```python
from build123d import *

# Parameters (mm, degrees)
SKETCH1_R           = 2.3
BOSS_EXTRUDE2_DEPTH = 4
FILLET1_R           = 4
FILLET2_R           = 30


with BuildPart() as part:
    # Sketch1 → Boss-Extrude2 (new body)
    with BuildSketch(Plane(origin=(0, 0, 0), x_dir=(1, 0, 0), z_dir=(0, 1, 0))):
        with BuildLine():
            Line((-4, -143.7), (-4, 4))
            Line((-4, 4), (25.4, 4))
            ThreePointArc((25.4, 4), (28.6800532, 2.289377864), (29.154640594, -1.379374498))
            Line((29.154640594, -1.379374498), (4, -69.85))
            Line((4, -69.85), (29.154640594, -138.320625502))
            ThreePointArc((29.154640594, -138.320625502), (28.6800532, -141.989377864), (25.4, -143.7))
            Line((25.4, -143.7), (-4, -143.7))
        make_face()
        with Locations(Location((0, 0, 0), (0, 0, 270))):
            Circle(SKETCH1_R, mode=Mode.SUBTRACT)
        with Locations(Location((25.4, 0, 0), (0, 0, 270))):
            Circle(SKETCH1_R, mode=Mode.SUBTRACT)
        with Locations(Location((25.4, -139.7, 0), (0, 0, 270))):
            Circle(SKETCH1_R, mode=Mode.SUBTRACT)
        with Locations(Location((0, -139.7, 0), (0, 0, 270))):
            Circle(SKETCH1_R, mode=Mode.SUBTRACT)
    extrude(amount=BOSS_EXTRUDE2_DEPTH)

    # Fillet1
    fillet1_edges = [part.edges().sort_by_distance(p)[0] for p in [
        (-4, 2, 143.7),
        (-4, 2, -4),
    ]]
    fillet(fillet1_edges, radius=FILLET1_R)

    # Fillet2
    fillet2_edges = [part.edges().sort_by_distance(p)[0] for p in [
        (4, 2, 69.85),
    ]]
    fillet(fillet2_edges, radius=FILLET2_R)


solid = part.part
```
Source: CAD feature listing. Evaluate the final solid. Frame: model axes, mm. A direction names the side the tool comes from. Round coordinates to 2 decimals unless told otherwise and drop trailing zeros. Loops run counter-clockwise (first coordinate to the right, second up) from the corner with the lowest first, then second, coordinate; pieces in that order, holes last.
1. Section query A-A on y = 3.15. Output: boundary loops of the cut face in (x, z), and give its area (3 significant figures).
2. Section query D-D on z = 127.5. Output: boundary loops of the cut face in (x, y), and give its area (3 significant figures).
3. Section query B-B on x = 10. Output: boundary loops of the cut face in (y, z), and give its area (3 significant figures).
4. Ray query, L1, parallel to X at y = 1.35, z = 0; L2, parallel to X at y = 0.2, z = 69; L3, parallel to X at y = 0.2, z = 78. Return the intervals inside material, ascending.
5. Access query for faces 4 (the cylindrical face through (-0.881, 1.972, 141.825)), 5 (the flat face through (18.328, 1.972, 108.851)). Directions: +Z, -Z, +X, -X, +Y, -Y. A direction counts if a zero-diameter tool reaches every point of the face in a straight line with its end or side. Return the directions, or none.
6. Contact query for a flat-ended pin moving along its axis: pin 1 (1.5 mm diameter, centred on y = 3, z = 50.5, fed in from +X). Output: stop coordinate, or through.
7. Mould query, pull axis Z, two halves, no side actions, for faces 1 (the cylindrical face through (24.519, 1.972, 141.825)), 2 (the cylindrical face through (-2.859, 2.028, -2.797)), 3 (the flat face through (13, 2, 143.7)). Classes: released by +Z, released by -Z, zero draft, split by the parting line, or undercut.
8. Section query C-C on z = 101. Output: boundary loops of the cut face in (x, y), and give its area (3 significant figures).
Answers below:
1. outline: (-4, 0) arc R4 ccw to (0, -4) - (25.4, -4) arc R4 ccw to (29.15, 1.38) - (7.8, 59.5) arc R30 cw to (7.8, 80.2) - (29.15, 138.32) arc R4 ccw to (25.4, 143.7) - (0, 143.7) arc R4 ccw to (-4, 139.7) - close; hole circle Ø4.6 at (0, 0); hole circle Ø4.6 at (0, 139.7); hole circle Ø4.6 at (25.4, 0); hole circle Ø4.6 at (25.4, 139.7)
1. area: 3,110 mm2
2. outline: (-4, 0) - (25.18, 0) - (25.18, 4) - (-4, 4) - close
2. area: 117 mm2
3. outline: (0, -4) - (4, -4) - (4, 53.52) - (0, 53.52) - close; (0, 86.18) - (4, 86.18) - (4, 143.7) - (0, 143.7) - close
3. area: 460 mm2
4. L1: x = -4 to -2.3, 2.3 to 23.1, 27.7 to 29.4
4. L2: x = -4 to 5.97
4. L3: x = -4 to 7.09
5. face 4: +Y, -Y
5. face 5: +X, +Y, -Y
6. pin 1: stops at x = 11.38
7. face 1: undercut
7. face 2: released by -Z
7. face 3: released by +Z
8. outline: (-4, 0) - (15.44, 0) - (15.44, 4) - (-4, 4) - close
8. area: 77.8 mm2
